For this review, take the finished solid that the model builds, in its own axes (mm). Face numbers are marked on the shaded views. A direction names the side the tool comes from. Round coordinates to 2 decimals unless told otherwise and drop trailing zeros. Order: outer loops, then holes, each group sorted by start corner. A loop starts at its lowest first (then second) coordinate and runs counter-clockwise, first axis right, second up. Notation, with made-up numbers: (15.5, 43) -> (60.5, 43) arc R27 ccw to (60.5, 63) -> close; hole circle Ø1 at (79.25, 10.5). An arc over 180 degrees is marked (long way). Use a Markdown table: item, result. Add a question column.
1) Consider section A-A (z = -1). State the section outline as (x, y) points, plus the area to 3 significant figures.
2) Wall thickness on line 1 along Z through (x, y) = (-22, 14.5); line 2 along Y through (x, z) = (-15.5, -3); line 3 along Z through (x, y) = (-8.5, -22.5): over which ranges is each line inside the solid? List them lowest first. Write a range as [from, to].
3) Draft analysis for pull direction Z (two halves, no side actions). For the marked faces 1, 2 and 3, state which applies: pulls with the +Z half, pulls with the -Z half, needs draft (parallel to the pull), parting line crosses it, or undercut.
4) Consider section C-C (x = -10.5). State the section outline as (y, z) points, plus the area to 3 significant figures.
5) Clearance check with flat-ended pins moving along their axes: P1, Ø2, axis at x = -30.5, y = -15.5, coming from the -Z side; P2, Ø15, axis at y = -14, z = -15, coming from the -X side; P3, Ø9, axis at y = -10, z = -9, coming from the +X side; P4, Ø10, axis at y = 17, z = -8, coming from the -X side. State where each tip first meets the part, or that it passes through.
6) Machinability: for the marked faces 4, 5 and 6, which of the approach directions +Z, -Z, +X, -X, +Y, -Y give a long, thin tool a straight path to every point of the face, cutting with its end or side? Answer none if there is none.
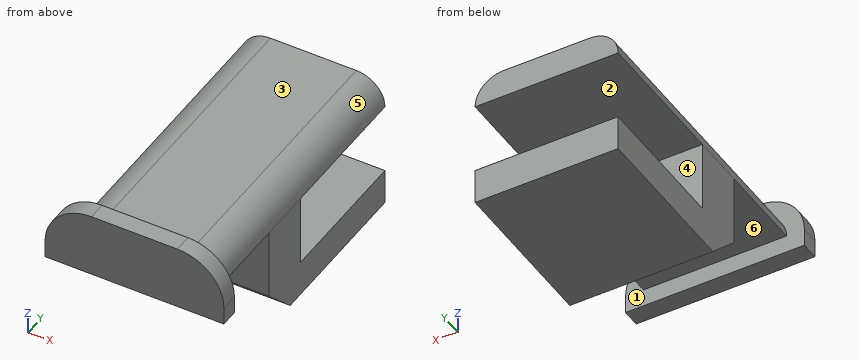
```python
from build123d import *

# Parameters (mm, degrees)
F0_W      = 40
F0_H      = 80
F1_DEPTH  = 8
F2_W      = 40
F2_H      = 15
F3_DEPTH  = 30
F4_W      = 40
F4_H      = 10
F5_DEPTH  = 40
F6_R      = 7.99999
F7_SIZE2  = 10
F7_SIZE   = 10
F9_DEPTH  = 5
F10_W     = 48
F10_H     = 5
F10_W_2   = 1
F11_DEPTH = 5


# Not quite as in the source:
# - a fillet or chamfer is up to 0.001 mm smaller than in the source, because OpenCascade refuses the exact size


with BuildPart() as f1:
    # F0 (on Top) → F1 (new body)
    with BuildSketch(Plane.XY):
        with Locations((-20, 2.0996452868)):
            Rectangle(F0_W, F0_H)
    extrude(amount=F1_DEPTH)

    # F2 (on face) → F3 (join)
    with BuildSketch(Plane(origin=(0, 0, 0), x_dir=(1, 0, 0), z_dir=(0, 0, -1))):
        with Locations((-20, 5.4003547132)):
            Rectangle(F2_W, F2_H)
    extrude(amount=F3_DEPTH)

    # F4 (on face) → F5 (join)
    with BuildSketch(Plane(origin=(0, 2.0996452868, 0), x_dir=(-1, 0, 0), z_dir=(0, 1, 0))):
        with Locations((20, -25)):
            Rectangle(F4_W, F4_H)
    extrude(amount=F5_DEPTH)

    # F6 (radius 8 in the source; OpenCascade refuses exactly that, so slightly less here)
    f6_edges = [f1.edges().sort_by_distance(p)[0] for p in [
        (0, 2.099645, 8),
        (-40, 2.099645, 8),
    ]]
    fillet(f6_edges, radius=F6_R)

    # F7
    f7_edges = [f1.edges().sort_by_distance(p)[0] for p in [
        (-20, -12.900355, -30),
    ]]
    chamfer(f7_edges, length=F7_SIZE, length2=F7_SIZE2)

    # F8 (on face) → F9 (join)
    with BuildSketch(Plane.XZ.offset(37.9003547132)):
        with BuildLine():
            Line((-44, -5), (4, -5))
            ThreePointArc((4, -5), (2.8166538264, 7.2111025509), (-8, 13))
            Line((-8, 13), (-32, 13))
            ThreePointArc((-32, 13), (-42.8166538264, 7.2111025509), (-44, -5))
        make_face()
    extrude(amount=F9_DEPTH)

    # F10 (on face) → F11 (join)
    with BuildSketch(Plane(origin=(0, 0, -5), x_dir=(1, 0, 0), z_dir=(0, 0, -1))):
        with Locations((-20, 40.4003547132)):
            Rectangle(F10_W, F10_H)
        with Locations((-44.5, 40.4003547132)):
            Rectangle(F10_W_2, F10_H)
        with Locations((4.5, 40.4003547132)):
            Rectangle(F10_W_2, F10_H)
    extrude(amount=-F11_DEPTH)


solid = f1.part
```
Results list:
| question | item | result |
|---|---|---|
| 1 | outline | (-45, -42.9) -> (5, -42.9) -> (5, -37.9) -> (-45, -37.9) -> close; (-40, -12.9) -> (0, -12.9) -> (0, 2.1) -> (-40, 2.1) -> close |
| 1 | area | 850 mm2 |
| 2 | line 1 | [-30, -20], [0, 8] |
| 2 | line 2 | [-42.9, -37.9], [-12.9, 2.1] |
| 2 | line 3 | [0, 8] |
| 3 | face 1 | needs draft |
| 3 | face 2 | undercut |
| 3 | face 3 | pulls with the +Z half |
| 4 | outline | (-42.9, -5) -> (-37.9, -5) -> (-37.9, 0) -> (-12.9, 0) -> (-12.9, -20) -> (-2.9, -30) -> (42.1, -30) -> (42.1, -20) -> (2.1, -20) -> (2.1, 0) -> (42.1, 0) -> (42.1, 8) -> (-37.9, 8) -> (-37.9, 13) -> (-42.9, 13) -> close |
| 4 | area | 1,530 mm2 |
| 5 | P1 | z = 0 |
| 5 | P2 | x = -40 |
| 5 | P3 | x = 0 |
| 5 | P4 | through |
| 6 | face 4 | +X, -X, +Y |
| 6 | face 5 | +Z, +X, +Y |
| 6 | face 6 | -Z, +X, -X |
